Work out the finished part from the listing and answer in its coordinate system (mm). Give positions to 0.01 mm unless a question says otherwise; leave off trailing zeros. Loops run counter-clockwise (first coordinate to the right, second up) from the corner with the lowest first, then second, coordinate; pieces in that order, holes last.
from build123d import *

# Parameters (mm, degrees)
SKETCH2_W                    = 77.55
SKETCH2_H                    = 1
F_10_0_1935_DIAMETER_HOLE1_D = 4.9149
CIRPATTERN3_COUNT            = 4
F_10_0_1935_DIAMETER_HOLE2_D = 4.9149


with BuildPart() as part:
    # Sketch2 → Revolve1 (revolve)
    with BuildSketch(Plane(origin=(0, 0, 0), x_dir=(0, 0, -1), z_dir=(1, 0, 0))):
        with Locations((-38.775, 0.5)):
            Rectangle(SKETCH2_W, SKETCH2_H)
    revolve(axis=Axis((0, -0.05, 0), (0, 1, 0)))

    # #10 (0.1935) Diameter Hole1 (through all)
    with Locations(Plane(origin=(0, 1, 0), x_dir=(1, 0, 0), z_dir=(0, 1, 0))):
        with Locations((-25.333643223, 61.160825052)):
            f_10_0_1935_diameter_hole1 = Hole(F_10_0_1935_DIAMETER_HOLE1_D / 2)

    # CirPattern3: #10 (0.1935) Diameter Hole1 ×4 about axis
    cirpattern3_axis = Axis((0, 0, 0), (0, 1, 0))
    for i in range(1, CIRPATTERN3_COUNT):
        add(f_10_0_1935_diameter_hole1.rotate(cirpattern3_axis, i * 360 / CIRPATTERN3_COUNT), mode=Mode.SUBTRACT)

    # #10 (0.1935) Diameter Hole2 (through all)
    with Locations(Plane(origin=(0, 1, 0), x_dir=(1, 0, 0), z_dir=(0, 1, 0))):
        with Locations((0, 0)):
            Hole(F_10_0_1935_DIAMETER_HOLE2_D / 2)


solid = part.part
Item 1: Find section A-A, the plane x = 0. Write down the section's boundary in (y, z).
Item 2: Find section B-B, the plane z = 0. Write down the section's boundary in (x, y), plus the area to 3 significant figures.
Item 3: Find section C-C, the plane y = 0.35. Write down the section's boundary in (x, z).
Item 4: Find section D-D, the plane z = -16. Write down the section's boundary in (x, y).
Item 5: Flat-ended cylindrical pins translate along their axes: pin 1 Ø4 at (x, z) = (61.16, -25.33) entering from +Y; pin 2 Ø6 at (x, z) = (4, -1.5) entering from -Y. Find the tip coordinate at first contact, or state that the pin passes through.
Item 6: Consider line 1 (X direction, y = 0.95, z = 59); line 2 (Z direction, x = 18.5, y = 0.6); line 3 (Z direction, x = -8.5, y = 0.15). Determine where each line is inside the solid, lowest interval first.
Item 7: Determine the mould class of faces 1 (the face through (23.29, 0.51, 73.97)), 2 (the face through (-16, 0, -1)), 3 (the face through (-1.13, 0.49, 2.18)) for opening direction Z: released by +Z, released by -Z, zero draft, split by the parting line, or undercut.
Ans:
1. outline: (0, -77.55) - (1, -77.55) - (1, -2.46) - (0, -2.46) - close; (0, 2.46) - (1, 2.46) - (1, 77.55) - (0, 77.55) - close
2. outline: (-77.55, 0) - (-2.46, 0) - (-2.46, 1) - (-77.55, 1) - close; (2.46, 0) - (77.55, 0) - (77.55, 1) - (2.46, 1) - close
2. area: 150 mm2
3. outline: circle Ø155.1 at (0, 0); hole circle Ø4.91 at (-61.16, 25.33); hole circle Ø4.91 at (-25.33, -61.16); hole circle Ø4.91 at (0, 0); hole circle Ø4.91 at (25.33, 61.16); hole circle Ø4.91 at (61.16, -25.33)
4. outline: (-75.88, 0) - (75.88, 0) - (75.88, 1) - (-75.88, 1) - close
5. pin 1: passes through
5. pin 2: stops at y = 0
6. line 1: x = -50.33 to 24.16, 26.5 to 50.33
6. line 2: z = -75.31 to 75.31
6. line 3: z = -77.08 to 77.08
7. face 1: split by the parting line
7. face 2: zero draft
7. face 3: undercut
